For this review, take the finished solid that the model builds, in its own axes (mm). Give positions to 0.01 mm unless a question says otherwise; leave off trailing zeros. Write each loop counter-clockwise with the first axis right and the second up, starting at its lowest first coordinate (ties: lowest second). Pieces come first, ordered by that corner, then holes. Notation, with made-up numbers: M -24,-23.75 L -5,-23.75 A26 cw -5,-9.75 Z; hole C -37,-32.75 d10. An arc over 180 degrees is marked long. Use one line per item in the form item = value. Start each with the question number.
Q1. Clearance check with flat-ended pins moving along their axes: pin 1 Ø4 at (y, z) = (4, -89) entering from +X; pin 2 Ø1 at (x, y) = (0.5, 35.5) entering from +Z; pin 3 Ø0.6 at (x, z) = (1, 1) entering from -Y; pin 4 Ø1 at (y, z) = (11, -15.5) entering from -X. State where each tip first meets the part, or that it passes through.
Q2. Consider section A-A on z = -49.25. Write out the cut boundary in (x, y).
Q3. Consider section B-B on y = 4. Write out the cut boundary in (x, z), and give its area (3 significant figures).
Q4. For probe 1 along Y at (x, z) = (0.45, -89); probe 2 along Z at (x, y) = (0.7, 4); probe 3 along Y at (x, z) = (0.4, -32.25), list the stretches that pass through material, from the lowest coordinate up. Write a range as [from, to].
Q5. Consider section D-D on z = -66.25. Write out the cut boundary in (x, y), and give its area (3 significant figures).
Q6. Consider section C-C on y = 22. Give the number of separate pieces and of enclosed holes in the cut face, and give its area (3 significant figures).
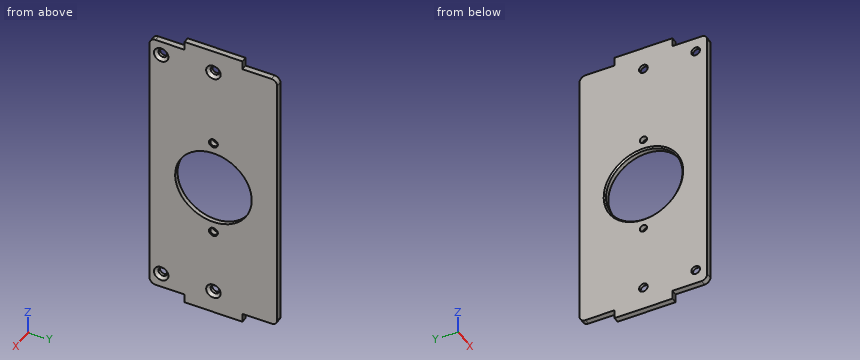
Autodesk Inventor part; units mm, degrees
ref_plane "YZ Plane" through (0, 0, 0) normal (1, 0, 0) x (0, 1, 0)
ref_plane "XZ Plane" through (0, 0, 0) normal (0, 1, 0) x (-1, 0, 0)
ref_plane "XY Plane" through (0, 0, 0) normal (0, 0, 1) x (1, 0, 0)
sketch "Sketch1" plane through (0, 0, 0) normal (1, 0, 0) x (0, 1, 0)
  line L0 (2, 0) -> (42, 0)
  line L1 (44, -2) -> (44, -92)
  line L2 (42, -94) -> (2, -94)
  line L3 (0, -92) -> (0, -2)
  line L4 (32, -94) -> (12, -94)
  line L5 (12, -94) -> (12, -97)
  line L6 (12, -97) -> (32, -97)
  line L7 (32, -97) -> (32, -94)
  line L8 (44.4582, -47) -> (27.4431, -47) construction
  line L9 (32, 0) -> (12, 0)
  line L10 (12, 0) -> (12, 3)
  line L11 (12, 3) -> (32, 3)
  line L12 (32, 3) -> (32, 0)
  arc A0 (42, -94) -> (44, -92) centre (42, -92) ccw
  arc A1 (0, -92) -> (2, -94) centre (2, -92) ccw
  arc A2 (2, 0) -> (0, -2) centre (2, -2) ccw
  arc A3 (44, -2) -> (42, 0) centre (42, -2) ccw
  point P0 (0, 0)
  point P1 (44, -94)
  point P2 (44, 0)
  point P3 (0, -94)
  point P4 (12, -95.5)
  point P5 (12, 1.5)
  dimension "d0" = 94
  dimension "d1" = 44
  dimension "d28" = 20
  dimension "d29" = 3
  dimension "d30" = 12
  dimension "d31" = 2
extrude "Extrusion1" add sketch "Sketch1" along normal blind 2
sketch "Sketch3" plane through (2, 0, 0) normal (1, 0, 0) x (0, 0, -1)
  circle A0 centre (49.25, 22) radius 13.2
  line L0 (0, 0) -> (92, 0)
  line L1 (94, 2) -> (94, 42)
  point P0 (120, 0)
  point P1 (120, 62)
  point P2 (94, 2)
  dimension "d23" = 26.4
  dimension "d24" = 22
  dimension "d25" = 44.75
extrude "Extrusion2" cut sketch "Sketch3" against normal through all
sketch "Sketch4" plane through (2, 0, 0) normal (1, 0, 0) x (0, 0, -1)
  circle A0 centre (5, 22) radius 1.5
  circle A1 centre (89, 22) radius 1.5
  line L0 (2, 0) -> (92, 0)
  line L1 (92, 44) -> (2, 44)
  line L2 (0, 42) -> (0, 32)
  line L3 (94, 32) -> (94, 42)
  circle A2 centre (89, 4) radius 1.5
  circle A3 centre (5, 4) radius 1.5
  point P0 (0, 0)
  dimension "d32" = 3
  dimension "d33" = 3
  dimension "d34" = 44
  dimension "d35" = 22
  dimension "d36" = 5
  dimension "d37" = 5
  dimension "d62" = 3
  dimension "d63" = 3
  dimension "d64" = 18
hole "Hole2" at (2, 22, -5) at (2, 22, -89) at (2, 4, -89) at (2, 4, -5) direction (-1, 0, 0) diameter 3 depth 14.2 tip angle 118
chamfer "Chamfer2" distance 1 angle 45 4 edges at (2, 4, -87.5) (2, 22, -87.5) (2, 4, -3.5) (2, 22, -3.5)
sketch "Sketch5" plane through (2, 0, 0) normal (1, 0, 0) x (0, 0, -1)
  circle A0 centre (66.25, 22) radius 1.5
  circle A1 centre (32.25, 22) radius 1.5
  circle A2 centre (89, 22) radius 1.5
  line L0 (89, 22) -> (83.0572, 22)
  circle A3 centre (49.25, 22) radius 13.2
  point P0 (0, 0)
  point P1 (49.25, 8.8)
  dimension "d48" = 3
  dimension "d49" = 3
  dimension "d50" = 34
  dimension "d51" = 17
hole "Hole3" at (2, 22, -66.25) at (2, 22, -32.25) direction (-1, 0, 0) diameter 2.459 depth 8.8 tip angle 118
chamfer "Chamfer3" distance 0.3 angle 45 2 edges at (2, 22, -65.0205) (2, 22, -31.0205)
chamfer "Chamfer4" distance 0.5 angle 45 1 edges at (0, 22, -36.05)
equation "\"d35\" = 0.5 * d34"
properties part number "ściana"
Working result:
q1.pin_1 = 1.5
q1.pin_2 = 0
q1.pin_3 = 12
q1.pin_4 = 0
q2.outline = M 0,0 L 2,0 L 2,8.8 L 0.5,8.8 L 0,8.3 Z; M 0,35.7 L 0.5,35.2 L 2,35.2 L 2,44 L 0,44 Z
q3.outline = M 0,-94 L 2,-94 L 2,-91.5 L 1,-90.5 L 0,-90.5 Z; M 0,-87.5 L 1,-87.5 L 2,-86.5 L 2,-7.5 L 1,-6.5 L 0,-6.5 Z; M 0,-3.5 L 1,-3.5 L 2,-2.5 L 2,0 L 0,0 Z
q3.area = 174 mm²
q4.probe_1 = [0, 2.5], [5.5, 20.5], [23.5, 44]
q4.probe_2 = [-94, -90.5], [-87.5, -6.5], [-3.5, 0]
q4.probe_3 = [0, 20.77], [23.23, 44]
q5.outline = M 0,0 L 2,0 L 2,20.47 L 1.7,20.77 L 0,20.77 Z; M 0,23.23 L 1.7,23.23 L 2,23.53 L 2,44 L 0,44 Z
q5.area = 83.0 mm²
q6.separate_pieces = 6
q6.enclosed_holes = 0
q6.area = 123 mm²
